Build history of the part. All positions in model axes, mm. Round coordinates to 2 decimals unless told otherwise and drop trailing zeros. Loops run counter-clockwise (first coordinate to the right, second up) from the corner with the lowest first, then second, coordinate; pieces in that order, holes last. Notation, with made-up numbers: (7, -35) -> (40, -35) arc R29 cw to (40, -7) -> close; hole circle Ø8 at (85, 5.25). An arc over 180 degrees is marked (long way). Put each result on its own line as item: value. Start each with the question number.
```python
from build123d import *

# Parameters (mm, degrees)
SK_P01_RECEIVER47X26X15_W  = 47
SK_P01_RECEIVER47X26X15_H  = 26
P01_RECEIVER47X26X15_DEPTH = 15
P02_ANTENNA_START          = 15
SK_P02_ANTENNA_R           = 0.8
P02_ANTENNA_DEPTH          = 22
P03_ANTENNA_START          = 15
SK_P03_ANTENNA_R           = 0.8
P03_ANTENNA_DEPTH          = 22


with BuildPart() as part:
    # SK_P01_Receiver47x26x15 → P01_Receiver47x26x15 (new body)
    with BuildSketch(Plane(origin=(0, 0, 0), x_dir=(1, 0, 0), z_dir=(0, 1, 0))):
        Rectangle(SK_P01_RECEIVER47X26X15_W, SK_P01_RECEIVER47X26X15_H)
    extrude(amount=P01_RECEIVER47X26X15_DEPTH)

    # SK_P02_Antenna → P02_Antenna (add)
    with BuildSketch(Plane(origin=(0, 0, 0), x_dir=(1, 0, 0), z_dir=(0, 1, 0)).offset(P02_ANTENNA_START)):
        with Locations(Location((-18.5, 9, 0), (0, 0, 270))):
            Circle(SK_P02_ANTENNA_R)
    extrude(amount=P02_ANTENNA_DEPTH)

    # SK_P03_Antenna → P03_Antenna (add)
    with BuildSketch(Plane(origin=(0, 0, 0), x_dir=(1, 0, 0), z_dir=(0, 1, 0)).offset(P03_ANTENNA_START)):
        with Locations(Location((-18.5, -9, 0), (0, 0, 270))):
            Circle(SK_P03_ANTENNA_R)
    extrude(amount=P03_ANTENNA_DEPTH)


solid = part.part
```
Item 1: Drop a flat-ended pin along its axis: pin 1 (4 mm diameter, centred on x = -1, z = 1.5, fed in from +Y). Give the stop position or say it passes through.
Item 2: Pull direction Z, two halves, no side cores. Call faces 1 (the face through (-18.99, 25.85, -9.63)), 2 (the face through (0, 7, 13)), 3 (the face through (23.5, 7, 0)), 4 (the face through (-19.28, 25.85, 8.83)): +Z half, -Z half, draft (parallel to the pull), parting line (faces both ways), or undercut.
Item 3: Cut at D-D on x = -13. Write the cut outline in (y, z), then the cut area to 3 significant figures.
Item 4: Cut at C-C on y = 33.5. Write the cut outline in (x, z).
Item 5: Cut at B-B on z = 9. Write the cut outline in (x, y).
Item 6: Cut at A-A on x = -18.5. Write the cut outline in (y, z).
Item 7: Wall check: line 1 (Y direction, x = 3, z = 6); line 2 (Z direction, x = -18, y = 16); line 3 (X direction, y = 24, z = -8.5). Give the ranges that are in metal, low to high. Write a range as from..to.
Ans:
1. pin 1: stops at y = 15
2. face 1: undercut
2. face 2: +Z half
2. face 3: draft
2. face 4: undercut
3. outline: (0, -13) -> (15, -13) -> (15, 13) -> (0, 13) -> close
3. area: 390 mm2
4. outline: circle Ø1.6 at (-18.5, -9); circle Ø1.6 at (-18.5, 9)
5. outline: (-23.5, 0) -> (23.5, 0) -> (23.5, 15) -> (-17.7, 15) -> (-17.7, 37) -> (-19.3, 37) -> (-19.3, 15) -> (-23.5, 15) -> close
6. outline: (0, -13) -> (15, -13) -> (15, -9.8) -> (37, -9.8) -> (37, -8.2) -> (15, -8.2) -> (15, 8.2) -> (37, 8.2) -> (37, 9.8) -> (15, 9.8) -> (15, 13) -> (0, 13) -> close
7. line 1: y = 0..15
7. line 2: z = -9.62..-8.38, 8.38..9.62
7. line 3: x = -19.12..-17.88
